```python
from build123d import *


with BuildPart() as part:
    # Sketch2 → Revolve1 (revolve)
    with BuildSketch(Plane(origin=(0, 0, 0), x_dir=(0, 0, -1), z_dir=(1, 0, 0))):
        with BuildLine():
            Line((0, 2.1), (0, 4))
            Line((0, 4), (-0.2, 4))
            ThreePointArc((-0.2, 4), (-0.5, 3.783772234), (-0.8, 4))
            Line((-0.8, 4), (-1, 4))
            Line((-1, 4), (-1, 2.1))
            Line((-1, 2.1), (0, 2.1))
        make_face()
    revolve1 = revolve(axis=Axis((0, 0, 3.014677367), (0, 0, -1)))

    # Mirror2: Revolve1 across plane
    add(revolve1.mirror(Plane(origin=(0, 0, 0), x_dir=(1, 0, 0), z_dir=(0, 0, -1))))


solid = part.part
```
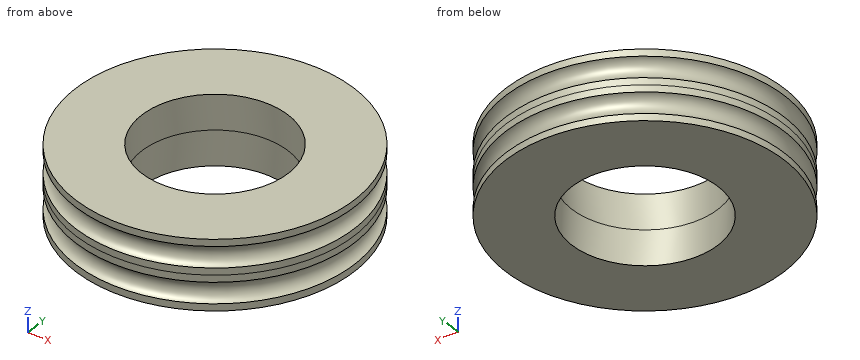
The listing builds one solid part. Answer for the finished solid, in the listing's coordinates (mm). Coordinates: 2 decimals unless noted, no trailing zeros. Loops run counter-clockwise (first coordinate to the right, second up) from the corner with the lowest first, then second, coordinate; pieces in that order, holes last. Notation, with made-up numbers: (56.25, 18.25) -> (114.25, 18.25) arc R17 ccw to (114.25, 47.25) -> close; hole circle Ø10 at (82.5, 25.25). An arc over 180 degrees is marked (long way). Use one line per item in the form item = value. Start each with the question number.
Item 1: Consider L1, parallel to X at y = 1, z = -0.6; L2, parallel to Y at x = -1.5, z = -0.75; L3, parallel to X at y = 1.5, z = -0.1. Determine where each line is inside the solid, lowest interval first. Write a range as [from, to].
Item 2: The part is cut by section D-D on z = -0.7. Determine the outline of the cut face in (x, y), then the cut area to 3 significant figures.
Item 3: The part is cut by section C-C on z = 0.1. Determine the outline of the cut face in (x, y), then the cut area to 3 significant figures.
Item 4: Flat-ended cylindrical pins translate along their axes: pin 1 Ø1 at (y, z) = (-1.5, 0.5) entering from +X; pin 2 Ø3.5 at (x, y) = (0, 0) entering from -Z. Find the tip coordinate at first contact, or state that the pin passes through.
Item 5: The part is cut by section A-A on y = 0. Determine the outline of the cut face in (x, z).
Answer key:
q1.L1 = [-3.67, -1.85], [1.85, 3.67]
q1.L2 = [-3.61, -1.47], [1.47, 3.61]
q1.L3 = [-3.71, -1.47], [1.47, 3.71]
q2.outline = circle Ø7.71 at (0, 0); hole circle Ø4.2 at (0, 0)
q2.area = 32.8 mm2
q3.outline = circle Ø8 at (0, 0); hole circle Ø4.2 at (0, 0)
q3.area = 36.4 mm2
q4.pin_1 = 3.85
q4.pin_2 = through
q5.outline = (-4, -1) -> (-2.1, -1) -> (-2.1, 1) -> (-4, 1) -> (-4, 0.8) arc R0.32 cw to (-4, 0.2) -> (-4, -0.2) arc R0.32 cw to (-4, -0.8) -> close; (2.1, -1) -> (4, -1) -> (4, -0.8) arc R0.32 cw to (4, -0.2) -> (4, 0.2) arc R0.32 cw to (4, 0.8) -> (4, 1) -> (2.1, 1) -> close
